from build123d import *

# Parameters (mm, degrees)
SKETCH_1_R      = 2.1
EXTRUDE_1_DEPTH = 60
SKETCH_2_R      = 2.1
EXTRUDE_2_DEPTH = 40


with BuildPart() as part:
    # 草图1 → 凸台-拉伸1 (new body)
    with BuildSketch(Plane(origin=(0, 0, 0), x_dir=(1, 0, 0), z_dir=(0, 1, 0))):
        Polygon((3.070700034, -1.603371853), (2.923910774, 1.85761831), (-0.14678926, 3.460990164), (-3.070700034, 1.603371853), (-2.923910774, -1.85761831), (0.14678926, -3.460990164), align=None)
        with Locations(Location((0, 0, 0), (0, 0, 270))):
            Circle(SKETCH_1_R, mode=Mode.SUBTRACT)
    extrude(amount=EXTRUDE_1_DEPTH)

    # 草图2 → 凸台-拉伸2 (add)
    with BuildSketch(Plane(origin=(0, 60, 0), x_dir=(1, 0, 0), z_dir=(0, 1, 0))):
        Polygon((-2.923910774, -1.85761831), (0.14678926, -3.460990164), (3.070700034, -1.603371853), (2.923910774, 1.85761831), (-0.14678926, 3.460990164), (-3.070700034, 1.603371853), align=None)
        with Locations(Location((0, 0, 0), (0, 0, 270))):
            Circle(SKETCH_2_R, mode=Mode.SUBTRACT)
    extrude(amount=EXTRUDE_2_DEPTH)


solid = part.part
Can you work these out from the model? Positions are in its coordinate system, mm. Round coordinates to 2 decimals unless told otherwise and drop trailing zeros. Order: outer loops, then holes, each group sorted by start corner. A loop starts at its lowest first (then second) coordinate and runs counter-clockwise, first axis right, second up. Notation, with made-up numbers: (52.5, 73.5) -> (109.5, 73.5) arc R25 cw to (109.5, 96.5) -> close; hole circle Ø9 at (77, -35). An arc over 180 degrees is marked (long way). Write each question's results on one line, items separated by ' | '. Start each with the question number.
Item 1: If we section it at C-C, the plane x = -1: Write out the boundary of the cut face in (y, z), then the cut area to 3 significant figures.
Item 2: Will these pins go through, and if not, where does the flat tip stop? pin 1 (1.5 mm diameter, centred on x = -1, y = 27.5, fed in from -Z); pin 2 (1 mm diameter, centred on y = 75.5, z = -2.5, fed in from +X); pin 3 (1.5 mm diameter, centred on x = 1, y = 15.5, fed in from +Z); pin 4 (2.5 mm diameter, centred on x = 0, z = 0, fed in from -Y).
Item 3: If we section it at B-B, the plane z = -0.25: Write out the boundary of the cut face in (x, y), then the cut area to 3 significant figures.
Item 4: If we section it at A-A, the plane y = 34: Write out the boundary of the cut face in (x, z).
Item 5: Please list where these lines run through material, in increasing order: L1, parallel to Z at x = 0.75, y = 16.5; L2, parallel to X at y = 28.5, z = 0; L3, parallel to Z at x = -1.5, y = 27.
Item 6: Thinking about a two-plate mould opening in X: for faces 1 (the flat face through (-3, 49.3, 0.1)), 2 (the cylindrical face through (0.631, 49.3, 2.003)), 3 (the flat face through (1.588, 49.3, 2.545)), which applies, +X half, -X half, draft (parallel to the pull), parting line (faces both ways), or undercut?
Results:
1) outline: (0, -2.92) -> (100, -2.92) -> (100, -1.85) -> (0, -1.85) -> close; (0, 1.85) -> (100, 1.85) -> (100, 2.86) -> (0, 2.86) -> close | area: 209 mm2
2) pin 1: stops at z = -3.4 | pin 2: stops at x = 2.65 | pin 3: stops at z = 3.4 | pin 4: passes through
3) outline: (-3.01, 0) -> (-2.09, 0) -> (-2.09, 100) -> (-3.01, 100) -> close; (2.09, 0) -> (2.99, 0) -> (2.99, 100) -> (2.09, 100) -> close | area: 184 mm2
4) outline: (-3.07, -1.6) -> (-0.15, -3.46) -> (2.92, -1.86) -> (3.07, 1.6) -> (0.15, 3.46) -> (-2.92, 1.86) -> close; hole circle Ø4.2 at (0, 0)
5) L1: z = -2.99 to -1.96, 1.96 to 3.08 | L2: x = -3 to -2.1, 2.1 to 3 | L3: z = -2.6 to -1.47, 1.47 to 2.6
6) face 1: -X half | face 2: undercut | face 3: +X half
